Read the model definition and answer for the solid it produces. Units are mm, in the model's axes. A direction names the side the tool comes from. Round coordinates to 2 decimals unless told otherwise and drop trailing zeros. Order: outer loops, then holes, each group sorted by start corner. A loop starts at its lowest first (then second) coordinate and runs counter-clockwise, first axis right, second up. Notation, with made-up numbers: M 44.25,63.5 L 101.25,63.5 A12 ccw 101.25,75.5 Z; hole C 70,12 d2. An arc over 180 degrees is marked long. Use one line per item in the form item = value. Start each with the question number.
from build123d import *

# Parameters (mm, degrees)
SKETCH1_W           = 105
SKETCH1_H           = 70
BOSS_EXTRUDE1_DEPTH = 5
SKETCH2_W           = 5
SKETCH2_H           = 70
BOSS_EXTRUDE2_DEPTH = 70
CUT_EXTRUDE1_DEPTH  = 20
SKETCH4_R           = 25.5
CUT_EXTRUDE2_DEPTH  = 10
BOSS_EXTRUDE3_DEPTH = 5
SKETCH6_R           = 25.5
SKETCH6_R_2         = 15.5
BOSS_EXTRUDE4_DEPTH = 5
SKETCH7_R           = 2.5
CUT_EXTRUDE3_DEPTH  = 5


with BuildPart() as part:
    # Sketch1 → Boss-Extrude1 (new body)
    with BuildSketch(Plane(origin=(0, 0, 0), x_dir=(1, 0, 0), z_dir=(0, 1, 0))):
        Rectangle(SKETCH1_W, SKETCH1_H)
    extrude(amount=BOSS_EXTRUDE1_DEPTH)

    # Sketch2 → Boss-Extrude2 (add)
    with BuildSketch(Plane(origin=(0, 5, 0), x_dir=(1, 0, 0), z_dir=(0, 1, 0))):
        with Locations((50, 0)):
            Rectangle(SKETCH2_W, SKETCH2_H)
    extrude(amount=BOSS_EXTRUDE2_DEPTH)

    # Sketch3 → Cut-Extrude1 (cut)
    with BuildSketch(Plane.ZY.offset(-47.5)):
        with BuildLine():
            Line((-18.027756377, 75), (-35, 75))
            Line((-35, 75), (-35, 45))
            ThreePointArc((-35, 45), (-30.462858313, 62.234101758), (-18.027756377, 75))
        make_face()
        with BuildLine():
            Line((35, 75), (18.027756377, 75))
            ThreePointArc((18.027756377, 75), (30.462858313, 62.234101758), (35, 45))
            Line((35, 45), (35, 75))
        make_face()
    extrude(amount=-CUT_EXTRUDE1_DEPTH, mode=Mode.SUBTRACT)

    # Sketch4 → Cut-Extrude2 (cut)
    with BuildSketch(Plane.ZY.offset(-47.5)):
        with Locations((0, 45)):
            Circle(SKETCH4_R)
    extrude(amount=-CUT_EXTRUDE2_DEPTH, mode=Mode.SUBTRACT)

    # Sketch5 → Boss-Extrude3 (add)
    with BuildSketch(Plane(origin=(52.5, 0, 0), x_dir=(0, 0, -1), z_dir=(1, 0, 0))):
        with BuildLine():
            Line((-18.027756377, 75), (18.027756377, 75))
            ThreePointArc((18.027756377, 75), (0, 80), (-18.027756377, 75))
        make_face()
    extrude(amount=-BOSS_EXTRUDE3_DEPTH)

    # Sketch6 → Boss-Extrude4 (add)
    with BuildSketch(Plane(origin=(52.5, 0, 0), x_dir=(0, 0, -1), z_dir=(1, 0, 0))):
        with Locations((0, 45)):
            Circle(SKETCH6_R)
        with Locations((0, 45)):
            Circle(SKETCH6_R_2, mode=Mode.SUBTRACT)
    extrude(amount=-BOSS_EXTRUDE4_DEPTH)

    # Sketch7 → Cut-Extrude3 (cut)
    with BuildSketch(Plane(origin=(52.5, 0, 0), x_dir=(0, 0, -1), z_dir=(1, 0, 0))):
        with Locations((14.142135624, 59.142135624)):
            Circle(SKETCH7_R)
        with Locations((14.142135624, 30.857864376)):
            Circle(SKETCH7_R)
        with Locations((-14.142135624, 30.857864376)):
            Circle(SKETCH7_R)
        with Locations((-14.142135624, 59.142135624)):
            Circle(SKETCH7_R)
    extrude(amount=-CUT_EXTRUDE3_DEPTH, mode=Mode.SUBTRACT)


solid = part.part
Item 1: Section D-D (z = -30) is taken. Write down the section's boundary in (x, y), and give its area (3 significant figures).
Item 2: Section B-B (x = 34.5) is taken. Write down the section's boundary in (y, z), and give its area (3 significant figures).
Item 3: A tool of negligible diameter and unlimited length cuts with its end or side. For faces 4 (the flat face through (-3, 5, 0)), 5 (the cylindrical face through (50.035, 28.417, 14.684)), from which of +Z, -Z, +X, -X, +Y, -Y can it reach the whole face along a straight path? Write none if from no direction.
Item 4: Section C-C (z = 21.5) is taken. Write down the section's boundary in (x, y), and give its area (3 significant figures).
Item 5: Given P1, Ø12, axis at y = 34.5, z = 13, coming from the -X side; P2, Ø1.5, axis at x = 14, z = -11.5, coming from the +Y side, each flat-ended and moving along its own axis, determine where each tip first touches the part or whether it passes through.
Item 6: Find the intervals of material crossed by L1, parallel to Y at x = 50.6, z = 0; L2, parallel to X at y = 64, z = -12; L3, parallel to Y at x = 32.5, z = 24, in increasing order. Write a range as [from, to].
Item 7: Section A-A (z = 0) is taken. Write down the section's boundary in (x, y).
Item 8: For a pull along Y with two mould halves and no side action, classify faces 1 (the cylindrical face through (50, 56.7, -13.6)), 2 (the flat face through (-1, 0, 0)), 3 (the flat face through (-52.5, 2, 0)) as pulls with the +Y half, pulls with the -Y half, needs draft (parallel to the pull), parting line crosses it, or undercut.
The answers:
q1.outline = M -52.5,0 L 52.5,0 L 52.5,63.03 L 47.5,63.03 L 47.5,5 L -52.5,5 Z
q1.area = 815 mm²
q2.outline = M 0,-35 L 5,-35 L 5,35 L 0,35 Z
q2.area = 350 mm²
q3.face_4 = +Z, -Z, -X, +Y
q3.face_5 = +X, -X
q4.outline = M -52.5,0 L 52.5,0 L 52.5,72.62 L 47.5,72.62 L 47.5,5 L -52.5,5 Z
q4.area = 863 mm²
q5.P1 = 47.5
q5.P2 = 5
q6.L1 = [0, 29.5], [60.5, 80]
q6.L2 = [47.5, 52.5]
q6.L3 = [0, 5]
q7.outline = M -52.5,0 L 52.5,0 L 52.5,29.5 L 47.5,29.5 L 47.5,5 L -52.5,5 Z; M 47.5,60.5 L 52.5,60.5 L 52.5,80 L 47.5,80 Z
q8.face_1 = undercut
q8.face_2 = pulls with the -Y half
q8.face_3 = needs draft
